The listing builds one solid part. Answer for the finished solid, in the listing's coordinates (mm). Face numbers are marked on the shaded views. Coordinates: 2 decimals unless noted, no trailing zeros. Loops run counter-clockwise (first coordinate to the right, second up) from the corner with the lowest first, then second, coordinate; pieces in that order, holes last. Notation, with made-up numbers: M 85,-6 L 140,-6 A26 cw 140,8 Z; hole C 27.5,-18.75 d8. An arc over 180 degrees is marked long. Answer in a Markdown table with one row per item. Add a question column.
Autodesk Inventor part; units mm, degrees
ref_plane "YZ Plane" through (0, 0, 0) normal (1, 0, 0) x (0, 1, 0)
ref_plane "XZ Plane" through (0, 0, 0) normal (0, 1, 0) x (-1, 0, 0)
ref_plane "XY Plane" through (0, 0, 0) normal (0, 0, 1) x (1, 0, 0)
sketch "Sketch1" plane through (0, 0, 0) normal (0, 1, 0) x (-1, 0, 0)
  line L0 (-40, 40) -> (40, 40)
  line L1 (40, 40) -> (40, -40)
  line L2 (40, -40) -> (-40, -40)
  line L3 (-40, -40) -> (-40, 40)
  line L4 (-40, 40) -> (40, -40) construction
  line L5 (40, 40) -> (-40, -40) construction
  line L6 (-25, 25) -> (25, 25) construction
  line L7 (25, 25) -> (25, -25) construction
  line L8 (25, -25) -> (-25, -25) construction
  line L9 (-25, -25) -> (-25, 25) construction
  line L10 (-25, 25) -> (25, -25) construction
  line L11 (25, 25) -> (-25, -25) construction
  circle A0 centre (0, 0) radius 10
  line L12 (20, 25) -> (-20, 25)
  line L13 (-20, 25) -> (-20, -25) construction
  line L14 (-20, -25) -> (20, -25) construction
  line L15 (20, -25) -> (20, 25) construction
  line L16 (56, 0) -> (-56, 0) construction
  line L17 (0, -56) -> (0, 56) construction
  dimension "d0" = 80
  dimension "d1" = 50
  dimension "d2" = 20
  dimension "d12" = 40
extrude "Extrusion1" add sketch "Sketch1" against normal blind 10
hole "Hole1" at (-25, 0, 25) at (25, 0, 25) at (-20, 0, -25) at (20, 0, -25) direction (0, -1, 0) diameter 8.376 end through all
chamfer "Chamfer1" distance 1 angle 45 8 edges at (20, 0, -29.188) (-20, 0, -29.188) (25, 0, 20.812) (-25, 0, 20.812) (20, -10, -29.188) (-20, -10, -29.188) (25, -10, 20.812) (-25, -10, 20.812)
chamfer "Chamfer2" distance 0.5 angle 45 2 edges at (10, 0, 0) (10, -10, 0)
properties part number "AP1-001"
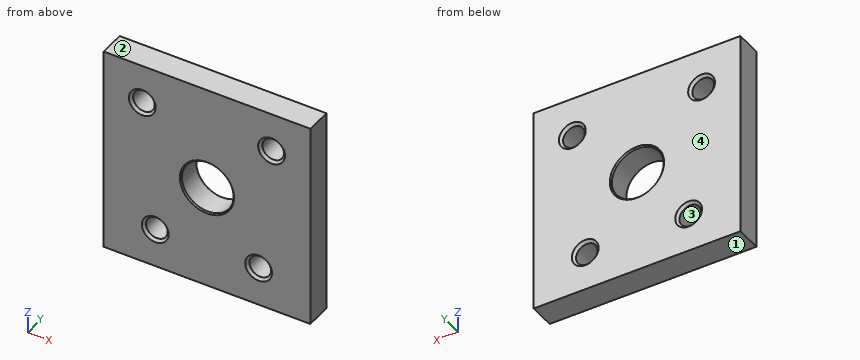
(1) The mould has two halves that part along Z. Classify the marked faces 1, 2, 3 and 4: released by +Z, released by -Z, zero draft, split by the parting line, or undercut.
(2) A cutting plane is placed at B-B (z = -25). Give the vertices of the cut face in (x, y), plus the area to 3 significant figures.
(3) A cutting plane is placed at A-A (x = 0). Give the vertices of the cut face in (y, z), plus the area to 4 significant figures.
(4) This flat-tipped pin is pushed along its axis until it touches: pin 1 (9.5 mm diameter, centred on x = 20, z = -25, fed in from -Y). Where does it stop, or does it pass through?
(5) Straight lines are drawn through the part: line 1 (X direction, y = -3.75, z = -25); line 2 (Z direction, x = 25, y = -6.5); line 3 (X direction, y = -4.25, z = 22). For each, find the intervals that lie inside material, in ascending order.
(6) A cutting plane is placed at C-C (y = -4). Give the vertices of the cut face in (x, z).
Solved:
| question | item | result |
|---|---|---|
| 1 | face 1 | released by -Z |
| 1 | face 2 | released by +Z |
| 1 | face 3 | undercut |
| 1 | face 4 | zero draft |
| 2 | outline | M -40,-10 L -25.19,-10 L -24.19,-9 L -24.19,-1 L -25.19,0 L -40,0 Z; M -15.81,-9 L -14.81,-10 L 14.81,-10 L 15.81,-9 L 15.81,-1 L 14.81,0 L -14.81,0 L -15.81,-1 Z; M 24.19,-9 L 25.19,-10 L 40,-10 L 40,0 L 25.19,0 L 24.19,-1 Z |
| 2 | area | 628 mm² |
| 3 | outline | M -10,-40 L 0,-40 L 0,-10.5 L -0.5,-10 L -9.5,-10 L -10,-10.5 Z; M -10,10.5 L -9.5,10 L -0.5,10 L 0,10.5 L 0,40 L -10,40 Z |
| 3 | area | 599.5 mm² |
| 4 | pin 1 | stops at y = -9.56 |
| 5 | line 1 | x = -40 to -24.19, -15.81 to 15.81, 24.19 to 40 |
| 5 | line 2 | z = -40 to 20.81, 29.19 to 40 |
| 5 | line 3 | x = -40 to -27.92, -22.08 to 22.08, 27.92 to 40 |
| 6 | outline | M -40,-40 L 40,-40 L 40,40 L -40,40 Z; hole C -25,25 d8.38; hole C -20,-25 d8.38; hole C 0,0 d20; hole C 20,-25 d8.38; hole C 25,25 d8.38 |
